Source: CAD feature listing. Evaluate the final solid. Frame: model axes, mm. Face numbers are marked on the shaded views. A direction names the side the tool comes from. Give positions to 0.01 mm unless a question says otherwise; leave off trailing zeros. Write each loop counter-clockwise with the first axis right and the second up, starting at its lowest first coordinate (ties: lowest second). Pieces come first, ordered by that corner, then holes. Notation, with made-up numbers: (4.25, -6) -> (36.25, -6) arc R27 ccw to (36.25, 24) -> close; hole circle Ø7 at (65, -21.5). An arc over 180 degrees is marked (long way). Use one line per item in the form item = value. Start each with the question number.
(1) Cut plane D-D, the plane x = 17.5. Output: boundary loops of the cut face in (y, z).
(2) Set-up query: the marked faces 3 and 4. Return all of +Z, -Z, +X, -X, +Y, -Y with unobstructed straight access to the full face (end or side cutting, diameter ignored); none if empty.
(3) Cut plane B-B, the plane y = -4.5. Output: boundary loops of the cut face in (x, z), and give its area (3 significant figures).
(4) Material intervals for line 1 along Z through (x, y) = (8, -0.75); line 2 along X through (y, z) = (-3.75, -1); line 3 along X through (y, z) = (-5.25, -19.5), sorted ascending. Write a range as from..to.
(5) Cut plane C-C, the plane z = -3. Output: boundary loops of the cut face in (x, y), and give its area (3 significant figures).
(6) Cut plane A-A, the plane z = 18. Output: boundary loops of the cut face in (x, y), and give its area (3 significant figures).
(7) First-contact query: P1, Ø5, axis at x = 18.5, z = -12.5, coming from the +Y side; P2, Ø1, axis at y = -2, z = 6.5, coming from the +X side; P3, Ø2, axis at x = -14.5, y = -3, coming from the -Z side. Flat tips, straight axial feed; report the tip coordinate or a pass-through.
(8) Draft query along Z for the marked faces 1 and 2. Return one class per face: pulls with the +Z half, pulls with the -Z half, needs draft (parallel to the pull), parting line crosses it, or undercut.
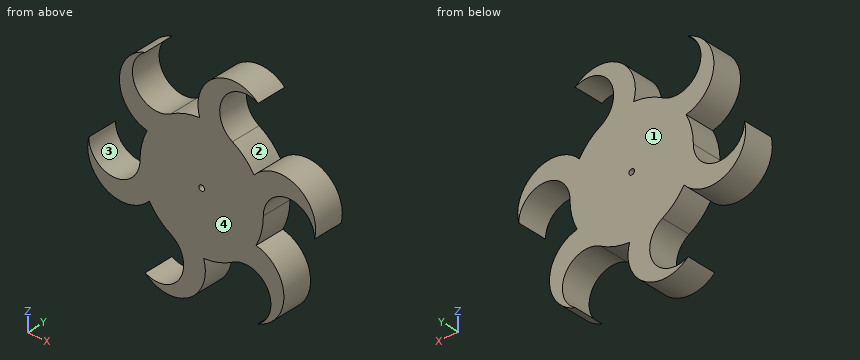
from build123d import *

# Parameters (mm, degrees)
F0_R     = 0.5715
F1_DEPTH = 6.35


with BuildPart() as f1:
    # F0 (on Front) → F1 (new body)
    with BuildSketch(Plane.XZ):
        with BuildLine():
            ThreePointArc((23.241, 0), (19.630978, 8.215892), (10.784784, 6.706597))
            ThreePointArc((10.784784, 6.706597), (8.832064, 9.126042), (6.35, 10.998523))
            ThreePointArc((6.35, 10.998523), (4.420863, 18.19816), (11.6205, 20.127296))
            ThreePointArc((11.6205, 20.127296), (2.700318, 21.108872), (-0.415691, 12.693195))
            ThreePointArc((-0.415691, 12.693195), (-3.487352, 12.211813), (-6.35, 10.998523))
            ThreePointArc((-6.35, 10.998523), (-13.549637, 12.92766), (-11.6205, 20.127296))
            ThreePointArc((-11.6205, 20.127296), (-16.93066, 12.89298), (-11.200475, 5.986598))
            ThreePointArc((-11.200475, 5.986598), (-12.319416, 3.085771), (-12.7, 0))
            ThreePointArc((-12.7, 0), (-17.9705, -5.2705), (-23.241, 0))
            ThreePointArc((-23.241, 0), (-19.630978, -8.215892), (-10.784784, -6.706597))
            ThreePointArc((-10.784784, -6.706597), (-8.832064, -9.126042), (-6.35, -10.998523))
            ThreePointArc((-6.35, -10.998523), (-4.420863, -18.19816), (-11.6205, -20.127296))
            ThreePointArc((-11.6205, -20.127296), (-2.700318, -21.108872), (0.415691, -12.693195))
            ThreePointArc((0.415691, -12.693195), (3.487352, -12.211813), (6.35, -10.998523))
            ThreePointArc((6.35, -10.998523), (13.549637, -12.92766), (11.6205, -20.127296))
            ThreePointArc((11.6205, -20.127296), (16.93066, -12.89298), (11.200475, -5.986598))
            ThreePointArc((11.200475, -5.986598), (12.319416, -3.085771), (12.7, 0))
            ThreePointArc((12.7, 0), (17.9705, 5.2705), (23.241, 0))
        make_face()
        Circle(F0_R, mode=Mode.SUBTRACT)
    extrude(amount=F1_DEPTH)


solid = f1.part
Geometry says:
q1.outline = (-6.35, 5.25) -> (0, 5.25) -> (0, 8.97) -> (-6.35, 8.97) -> close
q2.face_3 = +Y, -Y
q2.face_4 = +Z, -Z, +X, -X, -Y
q3.outline = (-23.24, 0) arc R7.29 ccw to (-10.78, -6.71) arc R12.7 ccw to (-6.35, -11) arc R5.27 cw to (-11.62, -20.13) arc R7.29 ccw to (0.42, -12.69) arc R12.7 ccw to (6.35, -11) arc R5.27 cw to (11.62, -20.13) arc R7.29 ccw to (11.2, -5.99) arc R12.7 ccw to (12.7, 0) arc R5.27 cw to (23.24, 0) arc R7.29 ccw to (10.78, 6.71) arc R12.7 ccw to (6.35, 11) arc R5.27 cw to (11.62, 20.13) arc R7.29 ccw to (-0.42, 12.69) arc R12.7 ccw to (-6.35, 11) arc R5.27 cw to (-11.62, 20.13) arc R7.29 ccw to (-11.2, 5.99) arc R12.7 ccw to (-12.7, 0) arc R5.27 cw to start; hole circle Ø1.14 at (0, 0)
q3.area = 790 mm^2
q4.line_1 = -10.39..9.86, 20.74..22.05
q4.line_2 = -23.42..-23.15, -12.8..12.66
q4.line_3 = -5.48..-0.87, 12.49..13.15
q5.outline = (-23.37, -6.35) -> (-22.3, -6.35) -> (-22.3, 0) -> (-23.37, 0) -> close; (-13.64, -6.35) -> (12.34, -6.35) -> (12.34, 0) -> (-13.64, 0) -> close
q5.area = 172 mm^2
q6.outline = (-15.05, -6.35) -> (-13.66, -6.35) -> (-13.66, 0) -> (-15.05, 0) -> close; (-0.07, -6.35) -> (4.31, -6.35) -> (4.31, 0) -> (-0.07, 0) -> close
q6.area = 36.7 mm^2
q7.P1 = 0
q7.P2 = 22.13
q7.P3 = -9.06
q8.face_1 = needs draft
q8.face_2 = undercut
